Input: part model. Units: mm. Frame: model coordinates. A direction names the side the tool comes from. Coordinates: 2 decimals unless noted, no trailing zeros. Order: outer loops, then holes, each group sorted by start corner. A loop starts at its lowest first (then second) coordinate and runs counter-clockwise, first axis right, second up. Notation, with made-up numbers: (23, 64) -> (42, 64) arc R29 ccw to (42, 86) -> close; hole circle Ø7 at (-19.5, -27). An arc over 180 degrees is marked (long way). Answer as CSV lines item,"result".
from build123d import *

# Parameters (mm, degrees)
BOSS_EXTRUDE1_DEPTH = 15
BOSS_EXTRUDE2_DEPTH = 60
CUT_EXTRUDE1_DEPTH  = 174.639610307
SCALE1_SCALE        = 0.3


with BuildPart() as part:
    # Sketch1 → Boss-Extrude1 (new body, symmetric)
    with BuildSketch(Plane.XY):
        Polygon((30, 0), (30, 100), (-33.639610307, 163.639610307), (-63.639610307, 163.639610307), (-63.639610307, 133.639610307), (-30, 66.606956932), (-30, 0), align=None)
    extrude(amount=BOSS_EXTRUDE1_DEPTH, both=True)

    # Sketch2 → Boss-Extrude2 (add)
    with BuildSketch(Plane(origin=(30, 0, 0), x_dir=(0, 0, -1), z_dir=(1, 0, 0))):
        Polygon((-15, -10), (15, -10), (6, 0), (-6, 0), align=None)
    extrude(amount=-BOSS_EXTRUDE2_DEPTH)

    # Sketch3 → Cut-Extrude1 (cut, through all)
    with BuildSketch(Plane(origin=(0, 163.639610307, 0), x_dir=(1, 0, 0), z_dir=(0, 1, 0))):
        Polygon((-63.639610307, 4.904583897), (-33.639610307, 15), (-33.639610307, 32.919088084), (-75.208668343, 32.919088084), (-75.208668343, 4.904583897), align=None)
        Polygon((-75.208668343, -32.919088084), (-75.208668343, -4.904583897), (-63.639610307, -4.904583897), (-33.639610307, -15), (-33.639610307, -32.919088084), align=None)
    extrude(amount=-CUT_EXTRUDE1_DEPTH, mode=Mode.SUBTRACT)


with BuildPart() as part_1:
    # Scale1: scaled about (-8.681688246, 73.036435377, 0)
    add(part.part.scale(SCALE1_SCALE).moved(Location((-6.077181772, 51.125504764, 0))))


solid = part_1.part
1. Reachability of faces 4 (the face through (-15.077, 60, 0)), 5 (the face through (-19.73, 89.93, -3.3)), 6 (the face through (-5.95, 49.65, 3.13)), 7 (the face through (-5.951, 49.605, -3.169)) from +Z, -Z, +X, -X, +Y, -Y: full face, straight path, thin tool, end or side. Return the list, or none.
Findings:
face 4,"+Z, -Z, -X, -Y"
face 5,"-Z, -X, +Y, -Y"
face 6,"+Z, +X, -X"
face 7,"-Z, +X, -X"
2. Cut plane A-A (z = -0.5). Return the cut outline in (x, y), plus the area to 3 significant figures.
Findings:
outline,"(-25.17, 91.22) -> (-15.08, 71.11) -> (-15.08, 48.13) -> (2.92, 48.13) -> (2.92, 81.13) -> (-16.17, 100.22) -> (-25.17, 100.22) -> close"
area,"948 mm2"
3. Cut plane D-D (x = 1). Return the cut outline in (y, z).
Findings:
outline,"(48.13, -4.5) -> (51.13, -1.8) -> (51.13, -4.5) -> (83.05, -4.5) -> (83.05, 4.5) -> (51.13, 4.5) -> (51.13, 1.8) -> (48.13, 4.5) -> close"
4. Cut plane C-C (y = 89). Return the cut outline in (x, z), plus the area to 3 significant figures.
Findings:
outline,"(-24.06, -1.85) -> (-16.17, -4.5) -> (-4.95, -4.5) -> (-4.95, 4.5) -> (-16.17, 4.5) -> (-24.06, 1.85) -> close"
area,"151 mm2"
5. Contact query for flat-ended pins moving along their axis: pin 1 (4.5 mm diameter, centred on y = 64, z = 2, fed in from -X); pin 2 (1 mm diameter, centred on y = 88.5, z = 1, fed in from -X). Output: stop coordinate, or through.
Findings:
pin 1,"stops at x = -15.08"
pin 2,"stops at x = -24.06"
6. Ray query, line 1 along X through (y, z) = (63, 2.5); line 2 along Y through (x, z) = (-14.5, 3.25); line 3 along Y through (x, z) = (-3.5, 3.25). Return the intervals inside material, ascending.
Findings:
line 1,"x = -15.08 to 2.92"
line 2,"y = 48.13 to 49.51, 51.13 to 98.55"
line 3,"y = 48.13 to 49.51, 51.13 to 87.55"
7. Mould query, pull axis Y, two halves, no side actions, for faces 1 (the face through (-6, 51.126, 3)), 2 (the face through (2.923, 64, 0)), 3 (the face through (-19.072, 79.069, 0.063)). Classes: released by +Y, released by -Y, zero draft, split by the parting line, or undercut.
Findings:
face 1,"undercut"
face 2,"zero draft"
face 3,"released by -Y"
8. Cut plane B-B (x = -8). Return the cut outline in (y, z).
Findings:
outline,"(48.13, -4.5) -> (51.13, -1.8) -> (51.13, -4.5) -> (92.05, -4.5) -> (92.05, 4.5) -> (51.13, 4.5) -> (51.13, 1.8) -> (48.13, 4.5) -> close"
